Read the model definition and answer for the solid it produces. Units are mm, in the model's axes. A direction names the side the tool comes from. Round coordinates to 2 decimals unless told otherwise and drop trailing zeros. Loops run counter-clockwise (first coordinate to the right, second up) from the corner with the lowest first, then second, coordinate; pieces in that order, holes last. Notation, with made-up numbers: (-24.75, 15.25) - (2.25, 15.25) arc R22 ccw to (2.25, 27.25) - close; hole circle Ø9 at (23.25, 67). An arc over 180 degrees is marked (long way). Use CSV: the item, a comma, the result in double quotes. Start each with the question number.
1. Find section C-C (z = 26). Give the vertices of the cut face in (x, y).
2. Find section B-B (x = 3). Give the vertices of the cut face in (y, z).
3. Determine the mould class of faces 1 (the flat face through (-15, 0, 236)), 2 (the flat face through (17.5, 0, 236)), 3 (the flat face through (0, 15, 236)), 4 (the flat face through (0, -17.5, 237)) for opening direction Y: +Y half, -Y half, draft (parallel to the pull), parting line (faces both ways), or undercut.
4. A tool of negligible diameter and unlimited length cuts with its end or side. For faces 5 (the flat face through (15, 0, 236)), 6 (the flat face through (0, 17.5, 236)), from which of +Z, -Z, +X, -X, +Y, -Y can it reach the whole face along a straight path? Write none if from no direction.
5. Find section A-A (y = 4.5). Give the vertices of the cut face in (x, z), and give its area (4 significant figures).
6. Given pin 1 Ø10 at (x, y) = (13.5, -7.5) entering from +Z, flat-ended and moving along its own axis, determine where the tip first touches the part or whether it passes through.
7. Consider line 1 along Y through (x, z) = (1, 317); line 2 along X through (y, z) = (-13, 377). Determine where each line is inside the solid, lowest interval first.
Autodesk Inventor part; units mm, degrees
ref_plane "Start plane" through (0, 0, -17.5) normal (0, 0, 1) x (1, 0, 0)
ref_plane "End plane" through (0, 0, 497.5) normal (0, 0, 1) x (1, 0, 0)
ref_plane "Work Plane4" through (17.5, 0, -17.5) normal (0, 0, -1) x (-1, 0, 0)
ref_plane "Start plane" through (0, 0, -17.5) normal (0, 0, 1) x (1, 0, 0)
ref_plane "End plane" through (0, 0, 497.5) normal (0, 0, 1) x (1, 0, 0)
sketch "Sketch" plane through (0, 0, 0) normal (0, 0, 1) x (1, 0, 0)
  line L0 (-17.5, -12.5) -> (-17.5, 12.5)
  line L1 (-12.5, 17.5) -> (12.5, 17.5)
  line L2 (17.5, 12.5) -> (17.5, -12.5)
  line L3 (12.5, -17.5) -> (-12.5, -17.5)
  arc A0 (-17.5, -12.5) -> (-12.5, -17.5) centre (-12.5, -12.5) ccw
  arc A1 (-12.5, 17.5) -> (-17.5, 12.5) centre (-12.5, 12.5) ccw
  arc A2 (17.5, 12.5) -> (12.5, 17.5) centre (12.5, 12.5) ccw
  arc A3 (12.5, -17.5) -> (17.5, -12.5) centre (12.5, -12.5) ccw
  arc A4 (-12.5, 15) -> (-15, 12.5) centre (-12.5, 12.5) ccw
  line L4 (-12.5, 15) -> (12.5, 15)
  arc A5 (15, 12.5) -> (12.5, 15) centre (12.5, 12.5) ccw
  line L5 (15, 12.5) -> (15, -12.5)
  arc A6 (12.5, -15) -> (15, -12.5) centre (12.5, -12.5) ccw
  line L6 (12.5, -15) -> (-12.5, -15)
  arc A7 (-15, -12.5) -> (-12.5, -15) centre (-12.5, -12.5) ccw
  line L7 (-15, -12.5) -> (-15, 12.5)
  line L8 (0, 25.9497) -> (0, -25.9497) construction
  line L9 (-25.9497, 0) -> (25.9497, 0) construction
  dimension "d7" = 5
  dimension "d10" = 35
  dimension "d11" = 35
  dimension "d12" = 2.5
  dimension "d15" = 17.5
  dimension "d16" = 17.5
extrude "Body" add sketch "Sketch" along normal up to surface (515 mm away) from surface at -17.5
sketch "Sketch3" plane through (0, 0, 0) normal (0, 0, 1) x (1, 0, 0)
  line L0 (0, 0) -> (10, 0)
ref_plane "Work Plane3" through (0, 0, 0) normal (0, -1, 0) x (1, 0, 0)
sketch "Sketch4" plane through (0, 0, 0) normal (0, -1, 0) x (1, 0, 0)
  line L0 (-2, -17.5) -> (12, -17.5)
  line L1 (-2, 497.5) -> (12, 497.5)
  dimension "d18" = 515
ref_plane "Work Plane4" through (17.5, 0, -17.5) normal (0, 0, -1) x (-1, 0, 0)
split "Split1" plane through (17.5, 0, -17.5) removes the side toward (0, 0, -1)
ref_plane "Work Plane5" through (0, 17.5, 497.5) normal (0, -0.7071, 0.7071) x (1, 0, 0)
split "Split2" plane through (0, 17.5, 497.5) removes the side toward (0, -0.7071, 0.7071)
ref_plane "Work Plane15" through (0, 17.5, -17.5) normal (0, -0.7071, -0.7071) x (1, 0, 0)
split "Split6" plane through (0, 17.5, -17.5) removes the side toward (0, -0.7071, -0.7071)
equation "\"d7\" = G_IR"
equation "\"d10\" = G_H"
equation "\"d11\" = G_W"
equation "\"d12\" = G_T"
equation "\"d15\" = 0.5 * d10"
equation "\"d16\" = 0.5 * d11"
equation "\"d3\" = G_L"
equation "\"G_W\" = 35"
equation "\"G_H\" = 35"
equation "\"G_T\" = 2.5"
equation "\"G_IR\" = 5"
equation "\"G_L\" = 535"
equation "\"G_OFFSET_START\" = 17.5"
equation "\"G_OFFSET_END\" = 17.5"
equation "\"d13\" = -G_OFFSET_START"
equation "\"d14\" = G_OFFSET_END + B_L"
properties part number "AS 1163 - C350L0 35x35x2.5 SHS - 535" material "Steel, Mild"
Filled sheet:
1,outline,"(-17.5, -12.5) arc R5 ccw to (-12.5, -17.5) - (12.5, -17.5) arc R5 ccw to (17.5, -12.5) - (17.5, 12.5) arc R5 ccw to (12.5, 17.5) - (-12.5, 17.5) arc R5 ccw to (-17.5, 12.5) - close; hole (-15, -12.5) arc R2.5 ccw to (-12.5, -15) - (12.5, -15) arc R2.5 ccw to (15, -12.5) - (15, 12.5) arc R2.5 ccw to (12.5, 15) - (-12.5, 15) arc R2.5 ccw to (-15, 12.5) - close"
2,outline,"(-17.5, 17.5) - (-15, 15) - (-15, 465) - (-17.5, 462.5) - close; (15, -15) - (17.5, -17.5) - (17.5, 497.5) - (15, 495) - close"
3,face 1,"undercut"
3,face 2,"draft"
3,face 3,"undercut"
3,face 4,"-Y half"
4,face 5,"+Z, -Z"
4,face 6,"+Z, -Z, +X, -X, +Y"
5,outline,"(-17.5, -4.5) - (-15, -4.5) - (-15, 484.5) - (-17.5, 484.5) - close; (15, -4.5) - (17.5, -4.5) - (17.5, 484.5) - (15, 484.5) - close"
5,area,"2,445 mm²"
6,pin 1,"stops at z = 477.27"
7,line 1,"y = -17.5 to -15, 15 to 17.5"
7,line 2,"x = -17.47 to -14.95, 14.95 to 17.47"
